Input: dimensioned drawing with shaded views. Units: mm. Origin: part minimum x, y, z. Round coordinates to 2 decimals unless told otherwise and drop trailing zeros. Loops run counter-clockwise (first coordinate to the right, second up) from the corner with the lowest first, then second, coordinate; pieces in that order, holes last. Notation, with made-up numbers: M -38,70 L -14,70 A28 cw -14,108 Z; hole C 72,-14 d2. An arc over 180 degrees is marked long. Put each result on its own line as item: value. Start each with the question number.
1) Section A-A on z = 30. Output: boundary loops of the cut face in (x, y), plus the area to 3 significant figures.
2) Line query: probe 1 along Y at (x, z) = (12.5, 13.5); probe 2 along Z at (x, y) = (40.5, 41.5); probe 3 along X at (y, z) = (86.65, 7.5). Output: solid intervals per line, ascending.
3) Pin query (flat end, axial travel): pin 1 (8 mm diameter, centred on x = 43.23, z = 48.2, fed in from -Y); pin 2 (4 mm diameter, centred on y = 67, z = 16.5, fed in from +X); pin 3 (1.5 mm diameter, centred on x = 29, y = 74.5, fed in from +Z); pin 4 (5 mm diameter, centred on y = 48, z = 43.5, fed in from -X). Return the tip coordinate at first contact, or that it passes through.
4) Section B-B on x = 8. State how many separate pieces and enclosed holes the cut face has, plus the area to 3 significant figures.
5) Draft query along Y for the marked faces 1, 2 and 3. Return one class per face: +Y half, -Y half, draft (parallel to the pull), parting line (faces both ways), or undercut.
6) Section C-C on y = 18. Output: boundary loops of the cut face in (x, z), plus the area to 3 significant figures.
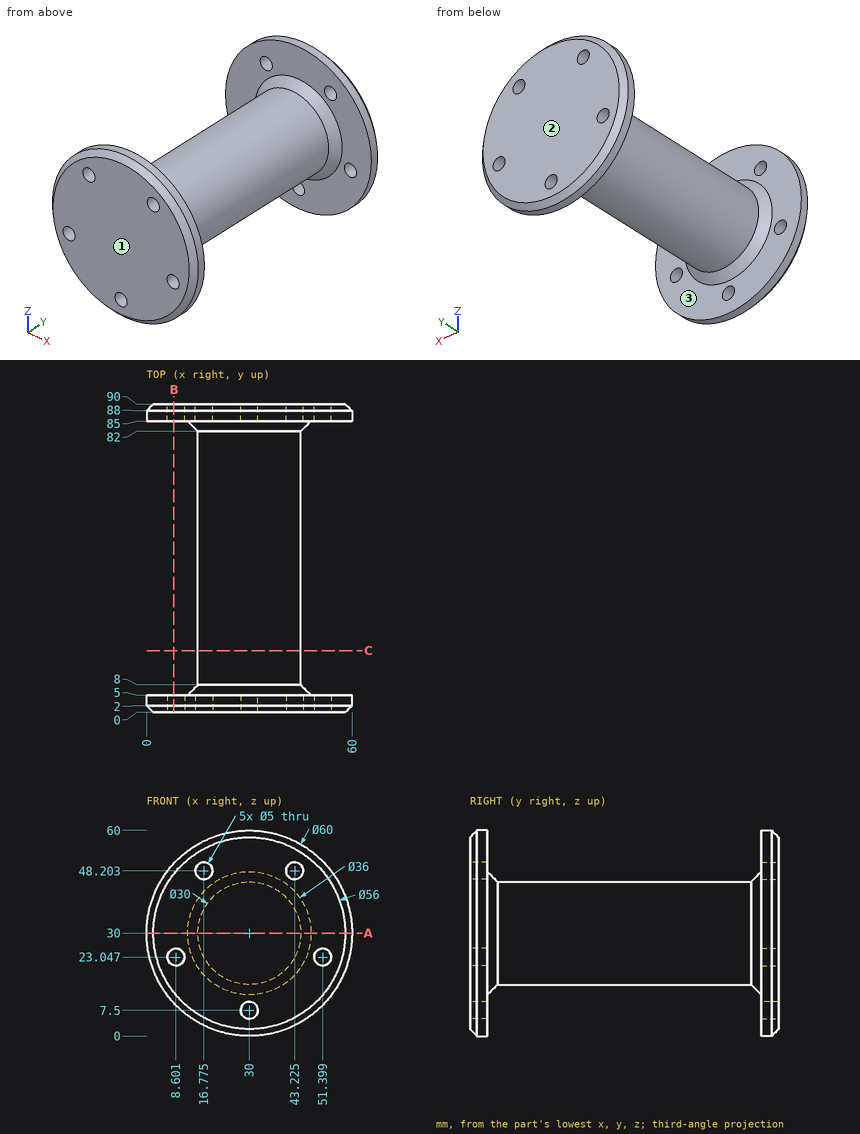
Geometry results:
1. outline: M 0,2 L 2,0 L 58,0 L 60,2 L 60,5 L 48,5 L 45,8 L 45,82 L 48,85 L 60,85 L 60,88 L 58,90 L 2,90 L 0,88 L 0,85 L 12,85 L 15,82 L 15,8 L 12,5 L 0,5 Z
1. area: 3,010 mm²
2. probe 1: y = 0 to 5, 85 to 90
2. probe 2: z = 19.29 to 40.71
2. probe 3: x = 10.16 to 27.5, 32.5 to 49.84
3. pin 1: stops at y = 0
3. pin 2: stops at x = 39.63
3. pin 3: stops at z = 45
3. pin 4: stops at x = 19.8
4. separate pieces: 4
4. enclosed holes: 0
4. area: 347 mm²
5. face 1: -Y half
5. face 2: +Y half
5. face 3: undercut
6. outline: C 30,30 d30
6. area: 707 mm²
